Design review of the part shown in the three views and the two pictorial views. Dimensions are in mm from the part's minimum x, y and z. A direction names the side the tool comes from. Round coordinates to 2 decimals unless told otherwise and drop trailing zeros. Loops run counter-clockwise (first coordinate to the right, second up) from the corner with the lowest first, then second, coordinate; pieces in that order, holes last. Notation, with made-up numbers: M -34.5,-15 L 6.5,-15 A23 ccw 6.5,18 Z; hole C -26,-28 d1. An arc over 180 degrees is marked long. Return JSON: item names as keys, results as strings. Group by question number.
Q1. Consider section A-A (y = 4). State the section outline as (x, z) points.
Q2. For the marked faces 1 and 2, list the 3-axis set-ups (+Z, -Z, +X, -X, +Y, -Y) from which the entire face can be reached by the end or side of a thin tool; tool diameter is ignored.
Q3. Consider section C-C (z = 1.25). State the section outline as (x, y) points.
Q4. Clearance check with flat-ended pins moving along their axes: pin 1 Ø3 at (y, z) = (2, 4.5) entering from -X; pin 2 Ø3 at (x, z) = (6.5, 4) entering from +Y. State where each tip first meets the part, or that it passes through.
Q5. Consider section D-D (y = 7.75). State the section outline as (x, z) points.
Q6. To check wall thickness, follow line 1 along Y through (x, z) = (4, 2.05); line 2 along X through (y, z) = (3, 1.45). State the ranges of each line that lie inside material, in increasing order.
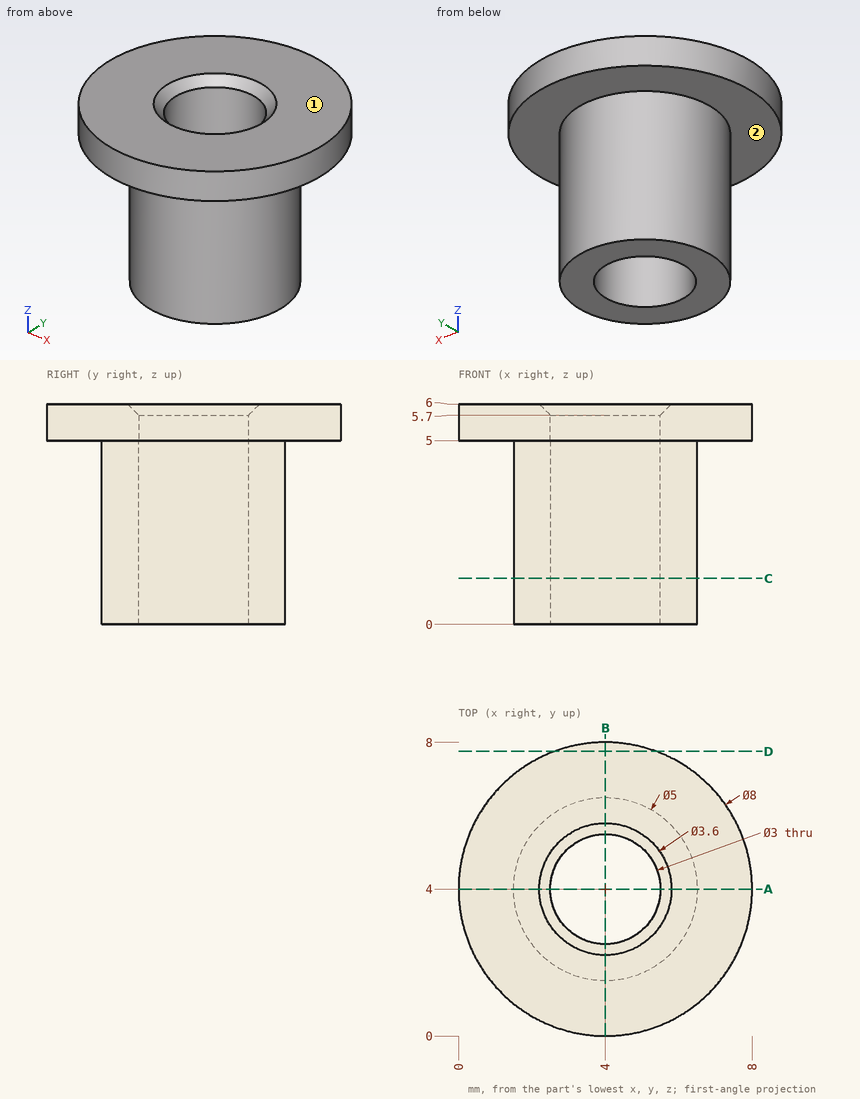
Values:
{
 "1": {"outline": "M 0,5 L 1.5,5 L 1.5,0 L 2.5,0 L 2.5,5.7 L 2.2,6 L 0,6 Z; M 5.5,0 L 6.5,0 L 6.5,5 L 8,5 L 8,6 L 5.8,6 L 5.5,5.7 Z"},
 "2": {"face 1": "+Z, +X, -X, +Y, -Y", "face 2": "-Z"},
 "3": {"outline": "C 4,4 d5; hole C 4,4 d3"},
 "4": {"pin 1": "stops at x = 0.04", "pin 2": "stops at y = 7.75"},
 "5": {"outline": "M 2.61,5 L 5.39,5 L 5.39,6 L 2.61,6 Z"},
 "6": {"line 1": "y = 1.5 to 2.5, 5.5 to 6.5", "line 2": "x = 1.71 to 2.88, 5.12 to 6.29"}
}
